The listing builds one solid part. Answer for the finished solid, in the listing's coordinates (mm). Face numbers are marked on the shaded views. A direction names the side the tool comes from. Give positions to 0.01 mm unless a question says otherwise; leave off trailing zeros. Loops run counter-clockwise (first coordinate to the right, second up) from the corner with the lowest first, then second, coordinate; pieces in that order, holes last. Notation, with made-up numbers: M 62,49 L 66,49 A28 ccw 66,87 Z; hole C 14,78.25 d2. An arc over 180 degrees is marked long. Use one line per item in the form item = value. Start each with the question number.
1. The part is cut by section C-C (z = 23.5). Write down the section's boundary in (x, y), and give its area (3 significant figures).
2. The part is cut by section B-B (x = -20). Write down the section's boundary in (y, z), and give its area (3 significant figures).
3. For the marked faces 1 and 2, determine the directions among +Z, -Z, +X, -X, +Y, -Y from which every point of the face is accessible in a straight line to the end or side of a thin tool.
4. The part is cut by section D-D (x = 16). Write down the section's boundary in (y, z).
5. Straight lines are drawn through the part: line 1 (X direction, y = -109, z = 16); line 2 (Z direction, x = -43.5, y = -50.5). For each, find the intervals that lie inside material, in ascending order. Write a range as from..to.
6. The part is cut by section A-A (y = -34.5). Write down the section's boundary in (x, z), and give its area (3 significant figures).
7. Each of these flat-tipped pins is pushed along its axis until it touches: pin 1 Ø11.5 at (x, y) = (-21.62, -115.96) entering from +Z; pin 2 Ø6 at (y, z) = (37.5, 36.5) entering from -X; pin 3 Ø6 at (x, y) = (41.71, 45.5) entering from +Z; pin 4 Ø16 at (x, y) = (41.71, -144.5) entering from +Z. Where does it stop, or does it pass through?
Autodesk Inventor part; units mm, degrees
ref_plane "YZ Plane" through (0, 0, 0) normal (1, 0, 0) x (0, 1, 0)
ref_plane "XZ Plane" through (0, 0, 0) normal (0, 1, 0) x (-1, 0, 0)
ref_plane "XY Plane" through (0, 0, 0) normal (0, 0, 1) x (1, 0, 0)
sketch "Sketch1" plane through (0, 0, 0) normal (0, 0, 1) x (1, 0, 0)
  line L0 (-52.5, 168.5) -> (52.5, 168.5)
  line L1 (52.5, 168.5) -> (52.5, -168.5)
  line L2 (52.5, -168.5) -> (-52.5, -168.5)
  line L3 (-52.5, -168.5) -> (-52.5, 168.5)
  line L4 (-52.5, 168.5) -> (52.5, -168.5) construction
  point P0 (0, 0)
  point P1 (0, 0)
  dimension "d0" = 105
  dimension "d1" = 337
extrude "Plate1" add sketch "Sketch1" along normal blind 2
sketch "Sketch4" plane through (50.5, 168.5, 0) normal (1, 0, 0) x (0, 1, 0)
  line L0 (-337, 0) -> (0, 0)
  line L1 (0, 0) -> (0, 45)
  line L2 (0, 45) -> (-337, 45)
  line L3 (-337, 45) -> (-337, 0)
edge flange "Flange1" height 45 angle 90 thickness 2 bend radius 2.75 thickness toward (1, 0, 0) relief round relief width 2 relief depth 1 edges at (52.5, 0, 2) wall of the first edge with corners at (50.5, -168.5, 0) (50.5, 168.5, 0) (50.5, 168.5, 45) (50.5, -168.5, 45)
bend "Bend1"
corner "Corner1"
sketch "Sketch5" plane through (0, 0, 0) normal (0, 0, -1) x (-1, 0, 0)
  line L0 (-47.75, 168.5) -> (-47.75, -168.5)
  line L1 (52.5, -168.5) -> (-47.75, -168.5)
  line L2 (52.5, 168.5) -> (52.5, -168.5)
  line L3 (-47.75, 168.5) -> (52.5, 168.5)
  line L4 (52.5, -168.5) -> (52.5, -179.0367)
  line L5 (-47.75, -168.5) -> (52.5, -168.5)
  line L6 (52.5, -179.0367) -> (-47.75, -168.5)
  point P0 (0, 0)
  dimension "d25" = 6
extrude "Extrusion2" add sketch "Sketch5" against normal up to surface (2 mm away) contours L1 L4 L6
sketch "Sketch6" plane through (0, 0, 0) normal (0, 0, -1) x (-1, 0, 0)
  line L0 (-47.75, 168.5) -> (-47.75, -168.5) construction
  line L1 (-47.75, -168.5) -> (52.5, -179.0367)
  line L2 (52.5, 168.5) -> (52.5, -179.0367)
  line L3 (-47.75, 168.5) -> (52.5, 168.5) construction
  line L4 (47.5274, -178.5141) -> (52.5, -131.2028)
  line L5 (-47.75, -168.5) -> (52.5, -179.0367)
  point P0 (0, 0)
  dimension "d29" = 5
extrude "Cut1" cut sketch "Sketch6" against normal blind 2
sketch "Sketch7" plane through (0, 0, 0) normal (0, 0, 1) x (1, 0, 0)
  line L0 (47.75, -168.5) -> (-47.5274, -178.5141)
  circle A0 centre (41.7082, -144.5001) radius 5.05
  line L1 (41.7082, -144.5001) -> (34.3912, -74.8835) construction
  line L2 (32.4201, -127.8799) -> (28.7616, -93.0716)
  circle A1 centre (34.3912, -74.8835) radius 5.05
  line L3 (-21.6216, -115.9635) -> (41.7082, -144.5001) construction
  line L4 (32.4201, -127.8799) -> (-6.0467, -96.7301) construction
  line L5 (28.7616, -93.0716) -> (-6.0467, -96.7301)
  line L6 (-2.3882, -131.5384) -> (32.4201, -127.8799)
  line L7 (28.7616, -93.0716) -> (-2.3882, -131.5384) construction
  line L8 (-6.0467, -96.7301) -> (-2.3882, -131.5384)
  line L9 (30.5908, -110.4758) -> (-21.6216, -115.9635) construction
  line L10 (34.3912, -74.8835) -> (-21.6216, -115.9635) construction
  circle A2 centre (-21.6216, -115.9635) radius 5.05
  point P0 (0, 0)
  point P1 (13.1867, -112.305)
  dimension "d32" = 35
  dimension "d33" = 35
  dimension "d34" = 10.1
  dimension "d35" = 70
  dimension "d36" = 60
  dimension "d37" = 25
  dimension "d38" = 11
  dimension "d39" = 42
extrude "Extrusion3" cut sketch "Sketch7" along normal through all
pattern_linear "Rectangular Pattern1" count 2 spacing 190 along (0, 1, 0) of "Extrusion3"
equation "\"d30\" = Thickness"
equation "\"d33\" = d32"
equation "\"d2\" = Thickness"
equation "\"d15\" = BendReliefWidth"
equation "\"d16\" = BendReliefDepth"
equation "\"d17\" = MinimumRemnant"
equation "\"d18\" = TransitionRadius"
equation "\"d21\" = BendRadius"
equation "\"d22\" = CornerReliefSize"
equation "\"d23\" = GapSize"
equation "\"d24\" = JacobiRadiusSize"
equation "\"BendReliefWidth\" = Thickness"
equation "\"BendReliefDepth\" = 0.5 * Thickness"
equation "\"CornerReliefSize\" = 4 * Thickness"
equation "\"MinimumRemnant\" = 2 * Thickness"
equation "\"TransitionRadius\" = BendRadius"
equation "\"JacobiRadiusSize\" = BendRadius"
equation "\"GapSize\" = Thickness"
properties part number "MNT-CDF-603 CAP" material "Stainless Steel"
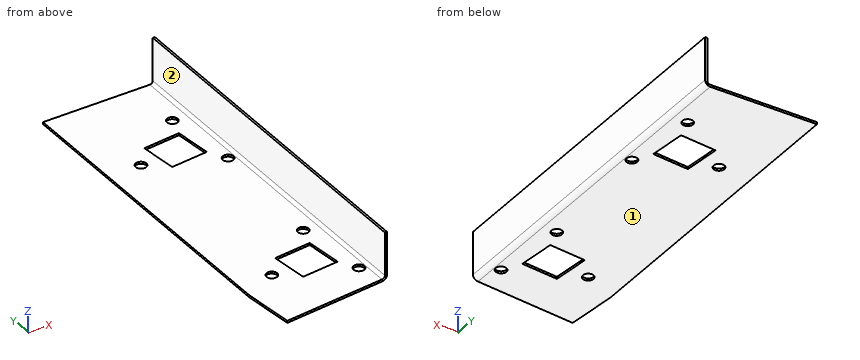
Derived:
q1.outline = M 50.5,-168.5 L 52.5,-168.5 L 52.5,168.5 L 50.5,168.5 Z
q1.area = 674 mm2
q2.outline = M -175.62,0 L -120.75,0 L -120.75,2 L -175.62,2 Z; M -111.18,0 L 69.25,0 L 69.25,2 L -111.18,2 Z; M 78.82,0 L 168.5,0 L 168.5,2 L 78.82,2 Z
q2.area = 650 mm2
q3.face_1 = -Z, +X, -X, +Y, -Y
q3.face_2 = +Z, -X, +Y, -Y
q4.outline = M -171.84,0 L -129.61,0 L -129.61,2 L -171.84,2 Z; M -94.41,0 L 60.39,0 L 60.39,2 L -94.41,2 Z; M 95.59,0 L 168.5,0 L 168.5,2 L 95.59,2 Z
q5.line_1 = 50.5..52.5
q5.line_2 = 0..2
q6.outline = M -52.5,0 L 47.75,0 A4.75 ccw 52.5,4.75 L 52.5,45 L 50.5,45 L 50.5,4.75 A2.75 cw 47.75,2 L -52.5,2 Z
q6.area = 293 mm2
q7.pin_1 = 2
q7.pin_2 = 50.5
q7.pin_3 = through
q7.pin_4 = 2.82
